For this review, take the finished solid that the model builds, in its own axes (mm). Round coordinates to 2 decimals unless told otherwise and drop trailing zeros. Answer as CSV lines item,"result". Start each with the question number.
Item 1: Mouldability with a two-part tool opening along Z and no side actions: class faces 1 (the flat face through (0, 10, 1)), 2 (the cylindrical face through (-0.568, 1.265, 32.032)), 3 (the cylindrical face through (38, 3, 0.4)) as +Z half, -Z half, draft (parallel to the pull), parting line (faces both ways), or undercut.
Item 2: For pin 1 Ø1.5 at (x, y) = (-22, 4.5) entering from -Z; pin 2 Ø3 at (y, z) = (3, 1.5) entering from -X; pin 3 Ø1.5 at (x, y) = (9, 7.5) entering from +Z; pin 4 Ø2.5 at (y, z) = (4.96, 0) entering from +X, all flat-tipped, find the tip position at first contact; note any pin that passes through.
Item 3: Wall thickness on probe 1 along Y at (x, z) = (39.5, 0); probe 2 along X at (y, z) = (7.5, 2); probe 3 along X at (y, z) = (2.25, -5): over which ranges is each line inside the solid? List them lowest first. Write a range as from..to.
```python
from build123d import *

# Parameters (mm, degrees)
SKETCH_1_W      = 100
SKETCH_1_H      = 70
EXTRUDE_1_DEPTH = 10
EXTRUDE_1_TAPER = 45
SKETCH_5_W      = 28.87382981
SKETCH_5_H      = 2
FILLET_1_R      = 2


with BuildPart() as part:
    # 草图1 → 凸台-拉伸1 (new body)
    with BuildSketch(Plane(origin=(0, 0, 0), x_dir=(1, 0, 0), z_dir=(0, 1, 0))):
        Rectangle(SKETCH_1_W, SKETCH_1_H)
    extrude(amount=EXTRUDE_1_DEPTH, taper=EXTRUDE_1_TAPER)

    # 草图2 one side → 切除-旋转2 (revolve, cut)
    with BuildSketch(Plane.XY):
        with BuildLine():
            ThreePointArc((21.414207954, 4.814992755), (25.414207954, 0.814992755), (29.414207954, 4.814992755))
            Line((29.414207954, 4.814992755), (21.414207954, 4.814992755))
        make_face()
    revolve(axis=Axis((65.414207954, 4.814992755, 0), (-1, 0, 0)), mode=Mode.SUBTRACT)

    # 草图5 → 切除-旋转4 (revolve, cut)
    with BuildSketch(Plane.XY, mode=Mode.PRIVATE) as cut_revolve_4_sk:
        with Locations((40.362985489, 5.961536801)):
            Rectangle(SKETCH_5_W, SKETCH_5_H)
    revolve(cut_revolve_4_sk.sketch.rotate(Axis((54.799900394, 4.961536801, 0), (-1, 0, 0)), 134.067661737), axis=Axis((54.799900394, 4.961536801, 0), (-1, 0, 0)), mode=Mode.SUBTRACT)

    # 圆角1
    # the kernel refuses this fillet: 2 mm, written as the material it takes off along each edge
    with BuildSketch(Plane(origin=(-62.071067812, 0, 35), x_dir=(0, 0.7071067811865464, -0.7071067811865487), z_dir=(1, 0, 0)), Plane(origin=(62.071067812, 0, -35), x_dir=(0, 0.7071067811865461, 0.707106781186549), z_dir=(-1, 0, 0))) as fillet_1_piece_1:
        with BuildLine():
            CenterArc((FILLET_1_R * 2.41421356237, -FILLET_1_R), FILLET_1_R, 90, 135)
            Line((FILLET_1_R * 1.70710678119, -FILLET_1_R * 1.70710678119), (0, 0))
            Line((0, 0), (FILLET_1_R * 2.41421356237, 0))
        make_face()
    extrude(amount=124.142135624, mode=Mode.SUBTRACT)
    with BuildSketch(Plane(origin=(-50, 0, -47.071067812), x_dir=(0.7071067811865483, 0.7071067811865466, 0), z_dir=(0, 0, 1)), Plane(origin=(50, 0, 47.071067812), x_dir=(-0.7071067811865485, 0.7071067811865467, 0), z_dir=(0, 0, -1))) as fillet_1_piece_2:
        with BuildLine():
            CenterArc((FILLET_1_R * 2.41421356237, -FILLET_1_R), FILLET_1_R, 90, 135)
            Line((FILLET_1_R * 1.70710678119, -FILLET_1_R * 1.70710678119), (0, 0))
            Line((0, 0), (FILLET_1_R * 2.41421356237, 0))
        make_face()
    extrude(amount=94.142135624, mode=Mode.SUBTRACT)


solid = part.part
```
Output values:
1,face 1,"draft"
1,face 2,"+Z half"
1,face 3,"undercut"
2,pin 1,"stops at z = -31.25"
2,pin 2,"stops at x = -47.17"
2,pin 3,"stops at z = 28.25"
2,pin 4,"stops at x = 21.67"
3,probe 1,"y = 0..2.96, 6.96..10"
3,probe 2,"x = -42.5..23.23, 27.6..42.5"
3,probe 3,"x = -47.16..47.16"
